from build123d import *

# Parameters (mm, degrees)
SKETCH_R     = 15
PAD_DEPTH    = 1
PAD001_DEPTH = 8
FILLET_R     = 2
CHAMFER_SIZE = 1


with BuildPart() as part:
    # Sketch → Pad (new body)
    with BuildSketch(Plane.XY):
        Circle(SKETCH_R)
    extrude(amount=-PAD_DEPTH)

    # Sketch001 → Pad001 (join)
    with BuildSketch(Plane.XY):
        with BuildLine():
            Line((-9.894317, 1.45), (9.894317, 1.45))
            ThreePointArc((9.996875, 0.25), (9.963678, 0.851545), (9.894317, 1.45))
            Line((9.996875, 0.25), (-9.996875, 0.25))
            ThreePointArc((-9.894317, 1.45), (-9.963678, 0.851545), (-9.996875, 0.25))
        make_face()
        with BuildLine():
            Line((-9.894317, -1.45), (9.894317, -1.45))
            ThreePointArc((9.894317, -1.45), (9.963678, -0.851545), (9.996875, -0.25))
            Line((9.996875, -0.25), (-9.996875, -0.25))
            ThreePointArc((-9.996875, -0.25), (-9.963678, -0.851545), (-9.894317, -1.45))
        make_face()
    extrude(amount=PAD001_DEPTH)

    # Fillet
    fillet_edges = [part.edges().sort_by_distance(p)[0] for p in [
        (9.963678, -0.851545, 8),
        (-9.963678, -0.851545, 8),
        (-9.963678, 0.851545, 8),
        (9.963678, 0.851545, 8),
    ]]
    fillet(fillet_edges, radius=FILLET_R)

    # Chamfer
    chamfer_edges = [part.edges().sort_by_distance(p)[0] for p in [
        (0, 1.45, 0),
        (0, -1.45, 0),
    ]]
    chamfer(chamfer_edges, length=CHAMFER_SIZE)


solid = part.part
Work out the finished part from the listing and answer in its coordinate system (mm). A direction names the side the tool comes from. Coordinates: 2 decimals unless noted, no trailing zeros. Write each loop counter-clockwise with the first axis right and the second up, starting at its lowest first coordinate (ties: lowest second). Pieces come first, ordered by that corner, then holes. Notation, with made-up numbers: M 43.5,-8.5 L 59.5,-8.5 A18 ccw 59.5,3.5 Z; hole C 1,42 d10. An arc over 180 degrees is marked long. Answer as CSV lines item,"result". Start each with the question number.
Item 1: Section A-A on z = 3.5 is taken. Write down the section's boundary in (x, y).
Item 2: Section B-B on x = 0 is taken. Write down the section's boundary in (y, z), and give its area (3 significant figures).
Item 3: Flat-ended cylindrical pins translate along their axes: P1, Ø12, axis at x = 10.5, y = 8, coming from the +Z side; P2, Ø4, axis at x = -3.5, z = 7, coming from the +Y side; P3, Ø2.5, axis at x = -1, z = 2, coming from the +Y side. Find the tip coordinate at first contact, or state that the pin passes through.
Item 4: Consider L1, parallel to Y at x = -7.25, z = 1; L2, parallel to Z at x = -12.25, y = 3.75. Determine where each line is inside the solid, lowest interval first.
Item 5: A tool of negligible diameter and unlimited length cuts with its end or side. For faces 1 (the face through (-9.96, 0.88, 2.96)), 2 (the face through (-9.964, -0.852, 2.958)), 3 (the face through (0, -1.45, 4)), from which of +Z, -Z, +X, -X, +Y, -Y can it reach the whole face along a straight path? Write none if from no direction.
Item 6: Section C-C on z = 6.75 is taken. Write down the section's boundary in (x, y).
Item 7: Section D-D on y = 12.5 is taken. Write down the section's boundary in (x, z), and give its area (3 significant figures).
Checks:
1,outline,"M -10,-0.25 A10 ccw -9.89,-1.45 L 9.89,-1.45 A10 ccw 10,-0.25 Z; M -10,0.25 L 10,0.25 A10 ccw 9.89,1.45 L -9.89,1.45 A10 ccw Z"
2,outline,"M -15,-1 L 15,-1 L 15,0 L 2.45,0 L 1.45,1 L 1.45,8 L 0.25,8 L 0.25,0 L -0.25,0 L -0.25,8 L -1.45,8 L -1.45,1 L -2.45,0 L -15,0 Z"
2,area,"50.2 mm²"
3,P1,"stops at z = 0.41"
3,P2,"stops at y = 1.45"
3,P3,"stops at y = 1.7"
4,L1,"y = -1.45 to -0.25, 0.25 to 1.45"
4,L2,"z = -1 to 0"
5,face 1,"+Z, -X, +Y"
5,face 2,"+Z, -X, -Y"
5,face 3,"+Z, +X, -X, -Y"
6,outline,"M -9.85,-0.25 A9.85 ccw -9.75,-1.45 L 9.75,-1.45 A9.85 ccw 9.85,-0.25 Z; M -9.85,0.25 L 9.85,0.25 A9.85 ccw 9.75,1.45 L -9.75,1.45 A9.85 ccw Z"
7,outline,"M -8.29,-1 L 8.29,-1 L 8.29,0 L -8.29,0 Z"
7,area,"16.6 mm²"
